```python
from build123d import *

# Parameters (mm, degrees)
F1_DEPTH = 3


with BuildPart() as f1:
    # F0 (on Front) → F1 (new body)
    with BuildSketch(Plane.XZ):
        with BuildLine():
            ThreePointArc((-99.755909, -71.773679), (-98.964341, -74.039735), (-96.764458, -75))
            Line((-96.764458, -75), (-77.459412, -75))
            ThreePointArc((-77.459412, -75), (-75.557445, -74.320026), (-74.51767, -72.588348))
            Line((-74.51767, -72.588348), (-52.411652, 37.941742))
            ThreePointArc((-52.411652, 37.941742), (-47.212775, 46.600132), (-37.702941, 50))
            Line((-37.702941, 50), (65, 50))
            ThreePointArc((65, 50), (68.535534, 48.535534), (70, 45))
            Line((70, 45), (70, 40))
            ThreePointArc((70, 40), (72.487506, 31.727304), (79.125, 26.198392))
            ThreePointArc((79.125, 26.198392), (81.954539, 26.456215), (83.3, 28.958714))
            Line((83.3, 28.958714), (83.3, 50))
            Line((83.3, 50), (86.7, 50))
            Line((86.7, 50), (86.7, 28.958714))
            ThreePointArc((86.7, 28.958714), (88.045461, 26.456215), (90.875, 26.198392))
            ThreePointArc((90.875, 26.198392), (97.512494, 31.727304), (100, 40))
            Line((100, 40), (100, 50))
            Line((100, 50), (100, 60))
            ThreePointArc((100, 60), (95.606602, 70.606602), (85, 75))
            Line((85, 75), (-69.00419, 75))
            ThreePointArc((-69.00419, 75), (-71.12551, 74.12132), (-72.00419, 72))
            Line((-72.00419, 72), (-72.00419, 50))
            Line((-72.00419, 50), (-75.40419, 50))
            Line((-75.40419, 50), (-75.40419, 71.428027))
            ThreePointArc((-75.40419, 71.428027), (-76.635782, 73.8514), (-79.319347, 74.285034))
            ThreePointArc((-79.319347, 74.285034), (-86.518028, 69.293112), (-89.700815, 61.131607))
            Line((-89.700815, 61.131607), (-99.755909, -71.773679))
        make_face()
    extrude(amount=-F1_DEPTH)


solid = f1.part
```
Verification items for the finished model (mm, model axes). A direction names the side the tool comes from. Round coordinates to 2 decimals unless told otherwise and drop trailing zeros. Write each loop counter-clockwise with the first axis right and the second up, starting at its lowest first coordinate (ties: lowest second). Pieces come first, ordered by that corner, then holes.
1. Gauge pin test, flat ends, axial feed: P1, Ø0.9, axis at x = 34.5, y = 1.5, coming from the -Z side; P2, Ø1.5, axis at y = 1, z = 43, coming from the -X side; P3, Ø1.5, axis at x = -73.5, y = 2, coming from the +Z side. Record the tip position at first contact, or that the pin passes through.
2. Section check D-D on x = -7.5. Enter the section's corners in (y, z).
3. Draft check along X on faces 3 (the cylindrical face through (72.42, 1.48, 31.83)), 4 (the flat face through (-23, 3, 51)), 5 (the cylindrical face through (95.72, 1.48, 70.49)). Enter one of: +X half, -X half, draft (parallel to the pull), parting line (faces both ways), or undercut.
4. Scan lines: L1, parallel to X at y = 0.75, z = 29; L2, parallel to Z at x = 44, y = 0.6; L3, parallel to X at y = 2.35, z = 37. Record each from-to range of solid material in increasing order.
5. Section check C-C on y = 2.25. Enter the section's corners in (x, z) (3 decimals), plus the area to 3 significant figures.
6. Section check A-A on z = 54.5. Enter the section's corners in (x, y), plus the area to 3 significant figures.
7. Section check B-B on z = 31.5. Enter the section's corners in (x, y).
8. Access from +Z, -Z, +X, -X, +Y, -Y to the whole of each face (thin tool, end or side, straight path). Record for faces 1 (the cylindrical face through (-47.32, 1.48, 46.51)), 2 (the flat face through (-94.658, 1.479, -4.391)).
Answer:
1. P1: stops at z = 50
1. P2: stops at x = -91.13
1. P3: stops at z = 50
2. outline: (0, 50) - (3, 50) - (3, 75) - (0, 75) - close
3. face 3: undercut
3. face 4: draft
3. face 5: +X half
4. L1: x = -92.13 to -54.2, 74.8 to 83.3, 86.7 to 95.2
4. L2: z = 50 to 75
4. L3: x = -91.53 to -52.6, 70.3 to 83.3, 86.7 to 99.7
5. outline: (-99.756, -71.774) arc R3 ccw to (-96.764, -75) - (-77.459, -75) arc R3 ccw to (-74.518, -72.588) - (-52.412, 37.942) arc R15 cw to (-37.703, 50) - (65, 50) arc R5 cw to (70, 45) - (70, 40) arc R15 ccw to (79.125, 26.198) arc R3 ccw to (83.3, 28.959) - (83.3, 50) - (86.7, 50) - (86.7, 28.959) arc R3 ccw to (90.875, 26.198) arc R15 ccw to (100, 40) - (100, 60) arc R15 ccw to (85, 75) - (-69.004, 75) arc R3 ccw to (-72.004, 72) - (-72.004, 50) - (-75.404, 50) - (-75.404, 71.428) arc R3 ccw to (-79.319, 74.285) arc R15 ccw to (-89.701, 61.132) - close
5. area: 9,250 mm2
6. outline: (-90.2, 0) - (-75.4, 0) - (-75.4, 3) - (-90.2, 3) - close; (-72, 0) - (100, 0) - (100, 3) - (-72, 3) - close
6. area: 560 mm2
7. outline: (-91.94, 0) - (-53.7, 0) - (-53.7, 3) - (-91.94, 3) - close; (72.64, 0) - (83.3, 0) - (83.3, 3) - (72.64, 3) - close; (86.7, 0) - (97.36, 0) - (97.36, 3) - (86.7, 3) - close
8. face 1: -Z, +Y, -Y
8. face 2: +Z, -X, +Y, -Y
